```python
from build123d import *

# Parameters (mm, degrees)
ESQUISSE1_W             = 72
ESQUISSE1_H             = 5
BOSS_EXTRU_1_DEPTH      = 50
ESQUISSE2_R             = 15
ENL_V_MAT_EXTRU_1_DEPTH = 6
ESQUISSE5_R             = 1.5
ENL_V_MAT_EXTRU_4_DEPTH = 51


with BuildPart() as part:
    # Esquisse1 → Boss.-Extru.1 (new body)
    with BuildSketch(Plane.XY):
        with Locations((16.5, -47.5)):
            Rectangle(ESQUISSE1_W, ESQUISSE1_H)
    extrude(amount=BOSS_EXTRU_1_DEPTH)

    # Esquisse2 → Enlèv. mat.-Extru.1 (cut, through all)
    with BuildSketch(Plane(origin=(0, -45, 0), x_dir=(-1, 0, 0), z_dir=(0, 1, 0))):
        with Locations((-16.5, 25)):
            Circle(ESQUISSE2_R)
    extrude(amount=-ENL_V_MAT_EXTRU_1_DEPTH, mode=Mode.SUBTRACT)

    # Esquisse5 → Enlèv. mat.-Extru.4 (cut, through all)
    with BuildSketch(Plane.XY.offset(50)):
        with Locations((16.5, -47.5)):
            Circle(ESQUISSE5_R)
    extrude(amount=-ENL_V_MAT_EXTRU_4_DEPTH, mode=Mode.SUBTRACT)


solid = part.part
```
Geometry: final body of the model. Coordinates: model frame, mm. Round coordinates to 2 decimals unless told otherwise and drop trailing zeros. Order: outer loops, then holes, each group sorted by start corner. A loop starts at its lowest first (then second) coordinate and runs counter-clockwise, first axis right, second up. Notation, with made-up numbers: (-34, -35.75) - (23, -35.75) arc R18 cw to (23, -17.75) - close; hole circle Ø11 at (9, 56.5). An arc over 180 degrees is marked (long way). Use CSV: the item, a comma, the result in double quotes. Start each with the question number.
Q1. Mould query, pull axis X, two halves, no side actions, for faces 1 (the face through (16, -45.8, 50)), 2 (the face through (16.175, -48.964, 5.109)), 3 (the face through (52.5, -48, 25)), 4 (the face through (16.175, -48.964, 45.032)). Classes: +X half, -X half, draft (parallel to the pull), parting line (faces both ways), or undercut.
Q2. Section query B-B (y = -47.5). Return loops of the section in (x, z).
Q3. Section query D-D (x = 3.5). Return loops of the section in (y, z), and give its area (3 significant figures).
Q4. Material intervals for line 1 along X through (y, z) = (-47.15, 25.5); line 2 along Y through (x, z) = (16.5, 45.25); line 3 along X through (y, z) = (-47.5, 4.25), sorted ascending. Write a range as from..to.
Q5. Section query A-A (z = 16). Return loops of the section in (x, y).
Q6. Section query C-C (x = 16.5). Return loops of the section in (y, z).
Result set:
1,face 1,"draft"
1,face 2,"undercut"
1,face 3,"+X half"
1,face 4,"undercut"
2,outline,"(-19.5, 0) - (15, 0) - (15, 10.08) arc R15 cw to (15, 39.92) - (15, 50) - (-19.5, 50) - close; (18, 0) - (52.5, 0) - (52.5, 50) - (18, 50) - (18, 39.92) arc R15 cw to (18, 10.08) - close"
3,outline,"(-50, 0) - (-45, 0) - (-45, 17.52) - (-50, 17.52) - close; (-50, 32.48) - (-45, 32.48) - (-45, 50) - (-50, 50) - close"
3,area,"175 mm2"
4,line 1,"x = -19.5..1.51, 31.49..52.5"
4,line 2,"y = -50..-49, -46..-45"
4,line 3,"x = -19.5..15, 18..52.5"
5,outline,"(-19.5, -50) - (4.5, -50) - (4.5, -45) - (-19.5, -45) - close; (28.5, -50) - (52.5, -50) - (52.5, -45) - (28.5, -45) - close"
6,outline,"(-50, 0) - (-49, 0) - (-49, 10) - (-50, 10) - close; (-50, 40) - (-49, 40) - (-49, 50) - (-50, 50) - close; (-46, 0) - (-45, 0) - (-45, 10) - (-46, 10) - close; (-46, 40) - (-45, 40) - (-45, 50) - (-46, 50) - close"
